```python
from build123d import *

# Parameters (mm, degrees)
F0_W     = 102
F0_H     = 3
F1_DEPTH = 50
F2_R     = 1.55
F3_DEPTH = 3
F4_R     = 2.8
F4_R_2   = 1.55
F5_DEPTH = 2.2


with BuildPart() as f1:
    # F0 (on Front) → F1 (new body, symmetric)
    with BuildSketch(Plane.XZ):
        with Locations((-0.412815, 0.432225)):
            Rectangle(F0_W, F0_H)
    extrude(amount=F1_DEPTH, both=True)

    # F2 (on face) → F3 (cut, through all)
    with BuildSketch(Plane.XY.offset(1.932225)):
        with Locations((-47.212815, 40.8)):
            Circle(F2_R)
        with Locations((14.687185, 40.8)):
            Circle(F2_R)
        with Locations((14.687185, -36)):
            Circle(F2_R)
        with Locations((-47.212815, -36)):
            Circle(F2_R)
        with Locations((-48.232815, 35.73)):
            Circle(F2_R)
        with Locations((-48.232815, -8.72)):
            Circle(F2_R)
        with Locations((47.017185, -8.72)):
            Circle(F2_R)
        with Locations((47.017185, 35.73)):
            Circle(F2_R)
    extrude(amount=-F3_DEPTH, mode=Mode.SUBTRACT)

    # F4 (on face) → F5 (cut)
    with BuildSketch(Plane(origin=(0, 0, -1.067775), x_dir=(1, 0, 0), z_dir=(0, 0, -1))):
        with Locations((-47.212815, 36)):
            Circle(F4_R)
        with Locations((-47.212815, 36)):
            Circle(F4_R_2, mode=Mode.SUBTRACT)
        with Locations((14.687185, 36)):
            Circle(F4_R)
        with Locations((14.687185, 36)):
            Circle(F4_R_2, mode=Mode.SUBTRACT)
        with Locations((-47.212815, -40.8)):
            Circle(F4_R)
        with Locations((-47.212815, -40.8)):
            Circle(F4_R_2, mode=Mode.SUBTRACT)
        with Locations((14.687185, -40.8)):
            Circle(F4_R)
        with Locations((14.687185, -40.8)):
            Circle(F4_R_2, mode=Mode.SUBTRACT)
    extrude(amount=-F5_DEPTH, mode=Mode.SUBTRACT)


solid = f1.part
```
Geometry: final body of the model. Coordinates: model frame, mm. A direction names the side the tool comes from. Give positions to 0.01 mm unless a question says otherwise; leave off trailing zeros. Loops run counter-clockwise (first coordinate to the right, second up) from the corner with the lowest first, then second, coordinate; pieces in that order, holes last. Notation, with made-up numbers: (15.25, -0.5) - (63.25, -0.5) arc R28 ccw to (63.25, 23.5) - close; hole circle Ø4 at (75, 41). An arc over 180 degrees is marked (long way). Answer as CSV lines item,"result". Start each with the question number.
(1) Section query A-A (y = 35.73). Output: boundary loops of the cut face in (x, z), and give its area (3 significant figures).
(2) Mould query, pull axis X, two halves, no side actions, for faces 3 (the face through (-51.413, -1, 0)), 4 (the face through (-46, -34.8, 1.132)), 5 (the face through (-1, 50, 0)). Classes: +X half, -X half, draft (parallel to the pull), parting line (faces both ways), or undercut.
(3) Pin query (flat end, axial travel): P1, Ø1.7, axis at x = -47.5, y = 40.5, coming from the -Z side; P2, Ø4, axis at x = -47.21, y = 40.8, coming from the -Z side. Return the tip coordinate at first contact, or that it passes through.
(4) Reachability of faces 1 (the face through (50.587, -1, 0)), 2 (the face through (12.465, 42.504, 0.017)) from +Z, -Z, +X, -X, +Y, -Y: full face, straight path, thin tool, end or side. Return the list, or none.
(5) Ray query, line 1 along X through (y, z) = (35, 1.5); line 2 along X through (y, z) = (40.8, 0.6). Return the intervals inside material, ascending. Write a range as [from, to].
Worked answers:
1,outline,"(-51.41, -1.07) - (-49.78, -1.07) - (-49.78, 1.93) - (-51.41, 1.93) - close; (-46.68, -1.07) - (45.47, -1.07) - (45.47, 1.93) - (-46.68, 1.93) - close; (48.57, -1.07) - (50.59, -1.07) - (50.59, 1.93) - (48.57, 1.93) - close"
1,area,"287 mm^2"
2,face 3,"-X half"
2,face 4,"undercut"
2,face 5,"draft"
3,P1,"passes through"
3,P2,"stops at z = 1.13"
4,face 1,"+Z, -Z, +X, +Y, -Y"
4,face 2,"-Z"
5,line 1,"x = [-51.41, -49.6], [-46.87, 45.65], [48.38, 50.59]"
5,line 2,"x = [-51.41, -50.01], [-44.41, 11.89], [17.49, 50.59]"
